from build123d import *

# Parameters (mm, degrees)
SKETCH_W   = 52
SKETCH_H   = 140
SKETCH_R   = 14
SKETCH_R_2 = 2.5
SKETCH_R_3 = 6
PAD_DEPTH  = 6


with BuildPart() as part:
    # Sketch → Pad (new body)
    with BuildSketch(Plane.XY):
        Rectangle(SKETCH_W, SKETCH_H)
        Circle(SKETCH_R, mode=Mode.SUBTRACT)
        with Locations((-15, 23)):
            Circle(SKETCH_R_2, mode=Mode.SUBTRACT)
        with Locations((0, 23)):
            Circle(SKETCH_R_2, mode=Mode.SUBTRACT)
        with Locations((-15, -23)):
            Circle(SKETCH_R_2, mode=Mode.SUBTRACT)
        with Locations((0, -23)):
            Circle(SKETCH_R_2, mode=Mode.SUBTRACT)
        with Locations((-18, 40)):
            Circle(SKETCH_R_2, mode=Mode.SUBTRACT)
        with Locations((18, 40)):
            Circle(SKETCH_R_2, mode=Mode.SUBTRACT)
        with Locations((18, -40)):
            Circle(SKETCH_R_2, mode=Mode.SUBTRACT)
        with Locations((-18, -40)):
            Circle(SKETCH_R_2, mode=Mode.SUBTRACT)
        with Locations((1, 55)):
            Circle(SKETCH_R_3, mode=Mode.SUBTRACT)
        with Locations((1, -55)):
            Circle(SKETCH_R_3, mode=Mode.SUBTRACT)
        with Locations((-17, 55)):
            Circle(SKETCH_R_2, mode=Mode.SUBTRACT)
        with Locations((19, 55)):
            Circle(SKETCH_R_2, mode=Mode.SUBTRACT)
        with Locations((-17, -55)):
            Circle(SKETCH_R_2, mode=Mode.SUBTRACT)
        with Locations((19, -55)):
            Circle(SKETCH_R_2, mode=Mode.SUBTRACT)
    extrude(amount=PAD_DEPTH)


solid = part.part
Source: CAD feature listing. Evaluate the final solid. Frame: model axes, mm. Give positions to 0.01 mm unless a question says otherwise; leave off trailing zeros. Write each loop counter-clockwise with the first axis right and the second up, starting at its lowest first coordinate (ties: lowest second). Pieces come first, ordered by that corner, then holes. Notation, with made-up numbers: M 54.25,58 L 83.25,58 A9 cw 83.25,63 Z; hole C 70,89.25 d8. An arc over 180 degrees is marked long. Return JSON: item names as keys, results as strings. Group by question number.
1) Cut plane C-C, the plane y = 0. Output: boundary loops of the cut face in (x, z), then the cut area to 3 significant figures.
2) Cut plane D-D, the plane x = 5. Output: boundary loops of the cut face in (y, z), then the cut area to 3 significant figures.
3) Cut plane A-A, the plane y = -40. Output: boundary loops of the cut face in (x, z), then the cut area to 3 significant figures.
4) Cut plane B-B, the plane z = 2.8. Give the number of separate pieces and of enclosed holes in the cut face, then the cut area to 3 significant figures.
5) First-contact query: pin 1 Ø15.5 at (x, y) = (1, -55) entering from +Z; pin 2 Ø3 at (x, y) = (18, -40) entering from -Z. Flat tips, straight axial feed; report the tip coordinate or a pass-through.
6) Ray query, L1, parallel to Y at x = 5.5, z = 2.2; L2, parallel to Y at x = -2, z = 1.1; L3, parallel to Y at x = 1, z = 3.85. Return the intervals inside material, ascending.
7) Draft query along Y for faces 1 (the face through (0, 70, 3)), 2 (the face through (-20, 38.5, 3)), 3 (the face through (-26, -1, 3)). Return one class per face: released by +Y, released by -Y, zero draft, split by the parting line, or undercut.
Data:
{
 "1": {"outline": "M -26,0 L -14,0 L -14,6 L -26,6 Z; M 14,0 L 26,0 L 26,6 L 14,6 Z", "area": "144 mm²"},
 "2": {"outline": "M -70,0 L -59.47,0 L -59.47,6 L -70,6 Z; M -50.53,0 L -13.08,0 L -13.08,6 L -50.53,6 Z; M 13.08,0 L 50.53,0 L 50.53,6 L 13.08,6 Z; M 59.47,0 L 70,0 L 70,6 L 59.47,6 Z", "area": "576 mm²"},
 "3": {"outline": "M -26,0 L -20.5,0 L -20.5,6 L -26,6 Z; M -15.5,0 L 15.5,0 L 15.5,6 L -15.5,6 Z; M 20.5,0 L 26,0 L 26,6 L 20.5,6 Z", "area": "252 mm²"},
 "4": {"separate pieces": "1", "enclosed holes": "15", "area": "6,200 mm²"},
 "5": {"pin 1": "stops at z = 6", "pin 2": "passes through"},
 "6": {"L1": "y = -70 to -58.97, -51.03 to -12.87, 12.87 to 51.03, 58.97 to 70", "L2": "y = -70 to -60.2, -49.8 to -24.5, -21.5 to -13.86, 13.86 to 21.5, 24.5 to 49.8, 60.2 to 70", "L3": "y = -70 to -61, -49 to -25.29, -20.71 to -13.96, 13.96 to 20.71, 25.29 to 49, 61 to 70"},
 "7": {"face 1": "released by +Y", "face 2": "undercut", "face 3": "zero draft"}
}
